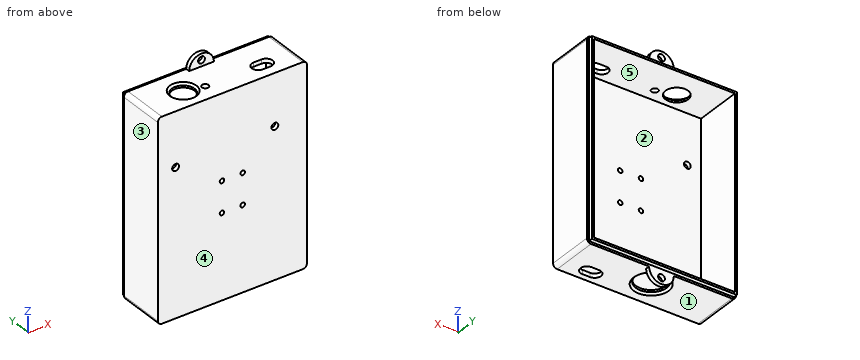
from build123d import *

# Parameters (mm, degrees)
BOSS_EXTRUDE1_DEPTH      = 18
BOSS_EXTRUDE1_DEPTH_BACK = 12.815459
SKETCH1_W                = 72.5
SKETCH1_H                = 96.828401578
SHELL1_T                 = 2
SKETCH2_R                = 7.5
CUT_EXTRUDE1_DEPTH       = 2
CHAMFER1_SIZE            = 1
SKETCH5_R                = 5.5
CUT_EXTRUDE2_DEPTH       = 2
CHAMFER2_SIZE            = 1
SKETCH8_W                = 72.5
SKETCH8_H                = 96.828401578
CUT_EXTRUDE5_DEPTH       = 8
BOSS_EXTRUDE3_START      = 10
SKETCH10_W               = 70.5
SKETCH10_H               = 94.828401578
SKETCH10_W_2             = 68.5
SKETCH10_H_2             = 92.828401578
BOSS_EXTRUDE3_DEPTH      = 2
CUT_EXTRUDE6_REACH       = 183.831
SKETCH12_R               = 1.6
FILLET1_R                = 2
BOSS_EXTRUDE4_START      = 10
SKETCH13_R               = 1.65
BOSS_EXTRUDE4_DEPTH      = 2
SKETCH16_R               = 1.65
BOSS_EXTRUDE5_DEPTH      = 2
SKETCH17_R               = 1.65
CUT_EXTRUDE8_DEPTH       = 12.81545914
SKETCH20_R               = 1.1
CUT_EXTRUDE9_DEPTH       = 2
CUT_EXTRUDE10_REACH      = 187.096
CUT_EXTRUDE11_REACH      = 187.096


with BuildPart() as part:
    # Sketch1 → Boss-Extrude1 (new, two sides: drawn at the far end of the back side and taken through both)
    with BuildSketch(Plane(origin=(0, 0, 0), x_dir=(1, 0, 0), z_dir=(0, 1, 0)).offset(-BOSS_EXTRUDE1_DEPTH_BACK)):
        with Locations((117.12025684, -15.018542133)):
            Rectangle(SKETCH1_W, SKETCH1_H)
    extrude(amount=BOSS_EXTRUDE1_DEPTH + BOSS_EXTRUDE1_DEPTH_BACK)

    # Shell1 (no face opened: a closed hollow body)
    add(offset(amount=-SHELL1_T, mode=Mode.PRIVATE), mode=Mode.SUBTRACT)

    # Sketch2 → Cut-Extrude1 (cut)
    with BuildSketch(Plane(origin=(0, 0, -33.395658656), x_dir=(-1, 0, 0), z_dir=(0, 0, -1))):
        with Locations((-114.89374317, -0.00045914)):
            Circle(SKETCH2_R)
    extrude(amount=-CUT_EXTRUDE1_DEPTH, mode=Mode.SUBTRACT)

    # Chamfer1
    chamfer1_edges = [part.edges().sort_by_distance(p)[0] for p in [
        (122.39374317, -0.00045914, -33.395658656),
    ]]
    chamfer(chamfer1_edges, length=CHAMFER1_SIZE)

    # Sketch5 → Cut-Extrude2 (cut)
    with BuildSketch(Plane.XY.offset(63.432742922)):
        with Locations((100.762134065, -2.34045914)):
            Circle(SKETCH5_R)
    extrude(amount=-CUT_EXTRUDE2_DEPTH, mode=Mode.SUBTRACT)

    # Chamfer2
    chamfer2_edges = [part.edges().sort_by_distance(p)[0] for p in [
        (95.262134065, -2.34045914, 63.432742922),
    ]]
    chamfer(chamfer2_edges, length=CHAMFER2_SIZE)

    # Sketch8 → Cut-Extrude5 (cut)
    with BuildSketch(Plane(origin=(0, 18, 0), x_dir=(1, 0, 0), z_dir=(0, 1, 0))):
        with Locations((117.12025684, -15.018542133)):
            Rectangle(SKETCH8_W, SKETCH8_H)
    extrude(amount=-CUT_EXTRUDE5_DEPTH, mode=Mode.SUBTRACT)

    # Sketch10 → Boss-Extrude3 (add)
    with BuildSketch(Plane(origin=(0, 0, 0), x_dir=(1, 0, 0), z_dir=(0, 1, 0)).offset(BOSS_EXTRUDE3_START)):
        with Locations((117.12025684, -15.018542133)):
            Rectangle(SKETCH10_W, SKETCH10_H)
        with Locations((117.12025684, -15.018542133)):
            Rectangle(SKETCH10_W_2, SKETCH10_H_2, mode=Mode.SUBTRACT)
    extrude(amount=BOSS_EXTRUDE3_DEPTH)

    # Sketch12 → Cut-Extrude6 (cut, up to next)
    with BuildSketch(Plane.XY.offset(63.432742922), mode=Mode.PRIVATE) as cut_extrude6_sk1:
        with Locations((109.796270245, -4.680244976)):
            Circle(SKETCH12_R)
    cut_extrude6_tool1 = extrude(cut_extrude6_sk1.sketch, amount=-CUT_EXTRUDE6_REACH, mode=Mode.PRIVATE) & part.part
    add(cut_extrude6_tool1.solids().sort_by_distance((109.79627, -4.680245, 63.432743))[0], mode=Mode.SUBTRACT)

    # Fillet1
    fillet1_edges = [part.edges().sort_by_distance(p)[0] for p in [
        (80.87025684, -1.4077295, -33.395658656),
        (153.37025684, -1.4077295, -33.395658656),
        (153.37025684, -1.4077295, 63.432742922),
        (80.87025684, -1.4077295, 63.432742922),
    ]]
    fillet(fillet1_edges, radius=FILLET1_R)

    # Sketch13 → Boss-Extrude4 (add)
    with BuildSketch(Plane(origin=(0, 0, 0), x_dir=(1, 0, 0), z_dir=(0, 1, 0)).offset(BOSS_EXTRUDE4_START)):
        with BuildLine():
            Line((111.12025684, -63.432742922), (123.12025684, -63.432742922))
            ThreePointArc((123.12025684, -63.432742922), (117.12025684, -69.432742922), (111.12025684, -63.432742922))
        make_face()
        with Locations(Location((117.12025684, -66.432742922, 0), (0, 0, 270))):
            Circle(SKETCH13_R, mode=Mode.SUBTRACT)
    boss_extrude4 = extrude(amount=-BOSS_EXTRUDE4_DEPTH)

    # Sketch16 → Boss-Extrude5 (add)
    with BuildSketch(Plane(origin=(0, 10, 0), x_dir=(1, 0, 0), z_dir=(0, 1, 0))):
        with BuildLine():
            Line((111.12025684, 33.395658656), (123.12025684, 33.395658656))
            ThreePointArc((123.12025684, 33.395658656), (117.12025684, 39.395658656), (111.12025684, 33.395658656))
        make_face()
        with Locations(Location((117.12025684, 36.395658656, 0), (0, 0, 270))):
            Circle(SKETCH16_R, mode=Mode.SUBTRACT)
    extrude(amount=-BOSS_EXTRUDE5_DEPTH)

    # Sketch17 → Cut-Extrude8 (cut)
    with BuildSketch(Plane(origin=(0, 0, 0), x_dir=(1, 0, 0), z_dir=(0, 1, 0))):
        with Locations(Location((137.785174065, -38.462742922, 0), (0, 0, 90))):
            Circle(SKETCH17_R)
        with Locations(Location((89.525174065, -37.192742922, 0), (0, 0, 90))):
            Circle(SKETCH17_R)
    extrude(amount=-CUT_EXTRUDE8_DEPTH, mode=Mode.SUBTRACT)

    # Mirror1: Boss-Extrude4 across plane
    add(boss_extrude4.mirror(Plane.XY.offset(15.018542133)))

    # Sketch20 → Cut-Extrude9 (cut)
    with BuildSketch(Plane.XZ.offset(12.81545914)):
        with Locations(Location((112.07025684, 22.518542133, 0), (0, 0, 270))):
            Circle(SKETCH20_R)
        with Locations(Location((122.17025684, 22.518542133, 0), (0, 0, 270))):
            Circle(SKETCH20_R)
        with Locations(Location((122.17025684, 7.518542133, 0), (0, 0, 270))):
            Circle(SKETCH20_R)
        with Locations(Location((112.07025684, 7.518542133, 0), (0, 0, 270))):
            Circle(SKETCH20_R)
    extrude(amount=-CUT_EXTRUDE9_DEPTH, mode=Mode.SUBTRACT)

    # Sketch21 → Cut-Extrude10 (cut, up to next)
    with BuildSketch(Plane.XY.offset(63.432742922), mode=Mode.PRIVATE) as cut_extrude10_sk1:
        with BuildLine():
            Line((139.29525684, -7.94045914), (135.44525684, -7.94045914))
            ThreePointArc((135.44525684, -7.94045914), (132.32025684, -4.81545914), (135.44525684, -1.69045914))
            Line((135.44525684, -1.69045914), (139.29525684, -1.69045914))
            ThreePointArc((139.29525684, -1.69045914), (142.42025684, -4.81545914), (139.29525684, -7.94045914))
        make_face()
    cut_extrude10_tool1 = extrude(cut_extrude10_sk1.sketch, amount=-CUT_EXTRUDE10_REACH, mode=Mode.PRIVATE) & part.part
    add(cut_extrude10_tool1.solids().sort_by_distance((137.370257, -4.815459, 63.432743))[0], mode=Mode.SUBTRACT)

    # Sketch23 → Cut-Extrude11 (cut, up to next)
    with BuildSketch(Plane(origin=(0, 0, -33.395658656), x_dir=(1, 0, 0), z_dir=(0, 0, -1)), mode=Mode.PRIVATE) as cut_extrude11_sk1:
        with BuildLine():
            Line((141.24525684, 3.69045914), (137.49525684, 3.69045914))
            ThreePointArc((137.49525684, 3.69045914), (134.37025684, 6.81545914), (137.49525684, 9.94045914))
            Line((137.49525684, 9.94045914), (141.24525684, 9.94045914))
            ThreePointArc((141.24525684, 9.94045914), (144.37025684, 6.81545914), (141.24525684, 3.69045914))
        make_face()
    cut_extrude11_tool1 = extrude(cut_extrude11_sk1.sketch, amount=-CUT_EXTRUDE11_REACH, mode=Mode.PRIVATE) & part.part
    add(cut_extrude11_tool1.solids().sort_by_distance((139.370257, -6.815459, -33.395659))[0], mode=Mode.SUBTRACT)


solid = part.part
Read the model definition and answer for the solid it produces. Units are mm, in the model's axes. Face numbers are marked on the shaded views. A direction names the side the tool comes from. Give positions to 0.01 mm unless a question says otherwise; leave off trailing zeros. Write each loop counter-clockwise with the first axis right and the second up, starting at its lowest first coordinate (ties: lowest second). Pieces come first, ordered by that corner, then holes. Notation, with made-up numbers: (16, -29) - (24, -29) arc R8 cw to (24, -17) - close; hole circle Ø10 at (-15.75, -11.75). An arc over 180 degrees is marked (long way). Use CSV: the item, a comma, the result in double quotes. Start each with the question number.
(1) Determine the mould class of the marked faces 1, 2 and 3 for opening direction Z: +Z half, -Z half, draft (parallel to the pull), parting line (faces both ways), or undercut.
(2) Given P1, Ø1.8, axis at x = 116.5, z = -37.5, coming from the -Y side; P2, Ø3, axis at x = 138.5, y = 6, coming from the +Z side; P3, Ø9, axis at x = 100.76, y = -2.34, coming from the +Z side, each flat-ended and moving along its own axis, determine where each tip first touches the part or whether it passes through.
(3) Find section A-A (x = 93). Give the vertices of the cut face in (y, z), plus the area to 3 significant figures.
(4) Find section B-B (z = -2). Give the vertices of the cut face in (x, y), plus the area to 3 significant figures.
(5) For the marked faces 4 and 5, determine the directions among +Z, -Z, +X, -X, +Y, -Y from which every point of the face is accessible in a straight line to the end or side of a thin tool.
(6) Consider line 1 along X through (y, z) = (9, -2); line 2 along Z through (x, y) = (88, 2); line 3 along X through (y, z) = (8.5, 61.5). Determine where each line is inside the solid, lowest interval first.
Findings below:
1,face 1,"-Z half"
1,face 2,"undercut"
1,face 3,"draft"
2,P1,"y = 8"
2,P2,"z = 63.43"
2,P3,"z = -31.4"
3,outline,"(-12.82, -33.4) - (10, -33.4) - (10, -32.4) - (12, -32.4) - (12, -31.4) - (-10.82, -31.4) - (-10.82, 61.43) - (12, 61.43) - (12, 62.43) - (10, 62.43) - (10, 63.43) - (-12.82, 63.43) - close"
3,area,"281 mm2"
4,outline,"(80.87, -12.82) - (153.37, -12.82) - (153.37, 10) - (152.37, 10) - (152.37, 12) - (151.37, 12) - (151.37, -10.82) - (82.87, -10.82) - (82.87, 12) - (81.87, 12) - (81.87, 10) - (80.87, 10) - close"
4,area,"232 mm2"
5,face 4,"+Z, -Z, +X, -X, -Y"
5,face 5,"+Y"
6,line 1,"80.87 to 82.87, 151.37 to 153.37"
6,line 2,"-33.4 to -31.4, 61.43 to 63.43"
6,line 3,"80.87 to 153.37"
